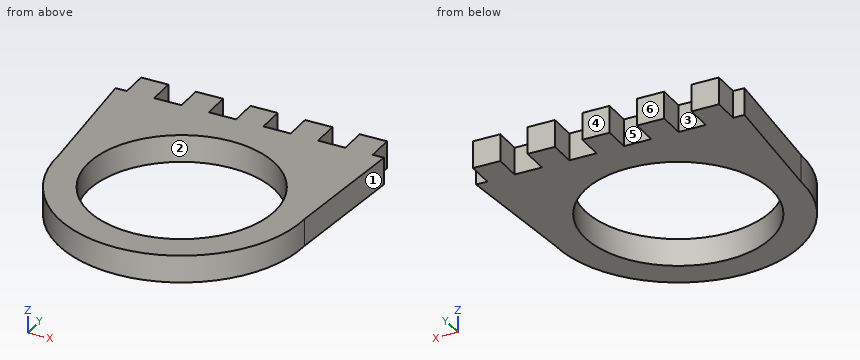
from build123d import *

# Parameters (mm, degrees)
BOSS_EXTRU_12_DEPTH        = 5
ESQUISSE4_R                = 17.05
ENL_V_MAT_EXTRU_1_DEPTH    = 5
ESQUISSE5_W                = 5
ESQUISSE5_H                = 5
ENL_V_MAT_EXTRU_2_DEPTH    = 10
R_P_TITION_LIN_AIRE1_COUNT = 4
R_P_TITION_LIN_AIRE1_PITCH = 10
ESQUISSE6_W                = 13.329947017
ESQUISSE6_H                = 14.257676648
ESQUISSE6_W_2              = 10.080555657
ESQUISSE6_H_2              = 33.311834117
ENL_V_MAT_EXTRU_3_DEPTH    = 10


with BuildPart() as part:
    # Esquisse3 → Boss.-Extru.12 (new body)
    with BuildSketch(Plane.XY):
        with BuildLine():
            Line((-22.5, 0), (-25, 28.75))
            Line((-25, 28.75), (25, 28.75))
            Line((25, 28.75), (22.5, 0))
            ThreePointArc((22.5, 0), (0, -22.5), (-22.5, 0))
        make_face()
    extrude(amount=BOSS_EXTRU_12_DEPTH)

    # Esquisse4 → Enlèv. mat.-Extru.1 (cut)
    with BuildSketch(Plane.XY.offset(5)):
        Circle(ESQUISSE4_R)
    extrude(amount=-ENL_V_MAT_EXTRU_1_DEPTH, mode=Mode.SUBTRACT)

    # Esquisse5 → Enlèv. mat.-Extru.2 (cut)
    with BuildSketch(Plane.XY.offset(5)):
        with Locations((-15, 26.25)):
            Rectangle(ESQUISSE5_W, ESQUISSE5_H)
    enl_v_mat_extru_2 = extrude(amount=-ENL_V_MAT_EXTRU_2_DEPTH, mode=Mode.SUBTRACT)

    # Répétition linéaire1: Enlèv. mat.-Extru.2 ×4
    with Locations(*[(i * R_P_TITION_LIN_AIRE1_PITCH, 0, 0) for i in range(1, R_P_TITION_LIN_AIRE1_COUNT)]):
        add(enl_v_mat_extru_2, mode=Mode.SUBTRACT)

    # Esquisse6 → Enlèv. mat.-Extru.3 (cut)
    with BuildSketch(Plane.XY.offset(5)):
        with Locations((29.164973509, 30.878838324)):
            Rectangle(ESQUISSE6_W, ESQUISSE6_H)
        with Locations((-27.540277829, 40.405917059)):
            Rectangle(ESQUISSE6_W_2, ESQUISSE6_H_2)
    extrude(amount=-ENL_V_MAT_EXTRU_3_DEPTH, mode=Mode.SUBTRACT)


solid = part.part
Check sheet for the modelled part. Datum: model origin and axes. Units: mm. Face numbers are marked on the shaded views. A direction names the side the tool comes from. Round coordinates to 2 decimals unless told otherwise and drop trailing zeros. Order: outer loops, then holes, each group sorted by start corner. A loop starts at its lowest first (then second) coordinate and runs counter-clockwise, first axis right, second up. Notation, with made-up numbers: M 27,24.25 L 36,24.25 A22 cw 36,44.25 Z; hole C 13,11 d10. An arc over 180 degrees is marked long. One line per item, written item: value. Start each with the question number.
1. Gauge pin test, flat ends, axial feed: P1, Ø1.5, axis at y = 25, z = 2.5, coming from the +X side; P2, Ø2.5, axis at x = -15, z = 3.5, coming from the +Y side; P3, Ø1.5, axis at y = 26.5, z = 3, coming from the -X side; P4, Ø2, axis at x = -9, y = -11, coming from the +Z side. Record the tip position at first contact, or that the pin passes through.
2. Section check C-C on y = 2. Enter the section's corners in (x, z), and give its area (3 significant figures).
3. Section check A-A on x = 0. Enter the section's corners in (y, z).
4. Scan lines: line 1 along Y through (x, z) = (0.5, 1.1); line 2 along X through (y, z) = (-0.5, 4.6); line 3 along Y through (x, z) = (-2, 3.15). Record each from-to range of solid material in increasing order.
5. Section check B-B on z = 2.4. Enter the section's corners in (x, y).
6. Section check D-D on y = -18. Enter the section's corners in (x, z), and give its area (3 significant figures).
7. Release check for a two-part mould opening along X. For the marked faces 1, 2, 3 and 4 record: released by +X, released by -X, zero draft, split by the parting line, or undercut.
8. Access from +Z, -Z, +X, -X, +Y, -Y to the whole of each face (thin tool, end or side, straight path). Record for the marked faces 5 and 6.
Results found:
1. P1: x = 22.5
1. P2: y = 23.75
1. P3: x = -22.5
1. P4: through
2. outline: M -22.67,0 L -16.93,0 L -16.93,5 L -22.67,5 Z; M 16.93,0 L 22.67,0 L 22.67,5 L 16.93,5 Z
2. area: 57.4 mm^2
3. outline: M -22.5,0 L -17.05,0 L -17.05,5 L -22.5,5 Z; M 17.05,0 L 28.75,0 L 28.75,5 L 17.05,5 Z
4. line 1: -22.49 to -17.04, 17.04 to 28.75
4. line 2: -22.49 to -17.04, 17.04 to 22.49
4. line 3: -22.41 to -16.93, 16.93 to 28.75
5. outline: M -24.57,23.75 L -22.5,0 A22.5 ccw 22.5,0 L 24.57,23.75 L 22.5,23.75 L 22.5,28.75 L 17.5,28.75 L 17.5,23.75 L 12.5,23.75 L 12.5,28.75 L 7.5,28.75 L 7.5,23.75 L 2.5,23.75 L 2.5,28.75 L -2.5,28.75 L -2.5,23.75 L -7.5,23.75 L -7.5,28.75 L -12.5,28.75 L -12.5,23.75 L -17.5,23.75 L -17.5,28.75 L -22.5,28.75 L -22.5,23.75 Z; hole C 0,0 d34.1
6. outline: M -13.5,0 L 13.5,0 L 13.5,5 L -13.5,5 Z
6. area: 135 mm^2
7. face 1: released by +X
7. face 2: undercut
7. face 3: undercut
7. face 4: zero draft
8. face 5: +Z, -Z, +Y
8. face 6: +Z, -Z, +X, -X, +Y
